Verification items for the finished model (mm, model axes). Give positions to 0.01 mm unless a question says otherwise; leave off trailing zeros. Loops run counter-clockwise (first coordinate to the right, second up) from the corner with the lowest first, then second, coordinate; pieces in that order, holes last. Notation, with made-up numbers: (40, 49) - (53, 49) arc R34 cw to (53, 81) - close; hole circle Ø1 at (26.25, 89). An arc over 180 degrees is marked (long way). Use one line per item in the form item = value.
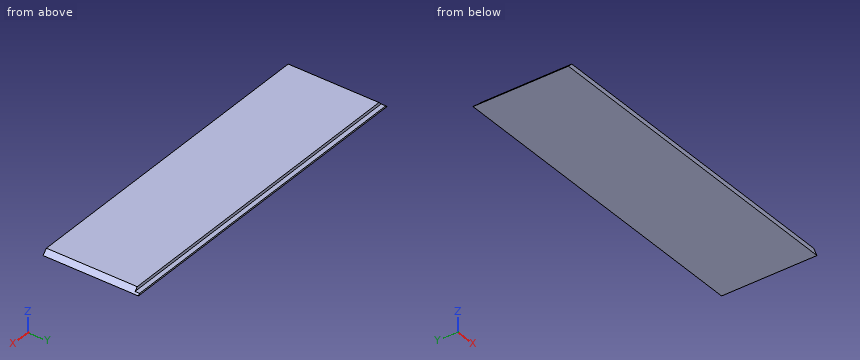
```python
from build123d import *

# Parameters (mm, degrees)
F0_W     = 1450
F0_H     = 415
F1_DEPTH = 20
F2_W     = 20
F2_H     = 13
F3_DEPTH = 1450
F5_DEPTH = 510


with BuildPart() as f1:
    # F0 (on Top) → F1 (new body)
    with BuildSketch(Plane.XY):
        Rectangle(F0_W, F0_H)
    extrude(amount=F1_DEPTH)

    # F2 (on face) → F3 (cut)
    with BuildSketch(Plane.YZ.offset(725)):
        with Locations((197.5, 13.5)):
            Rectangle(F2_W, F2_H)
    extrude(amount=-F3_DEPTH, mode=Mode.SUBTRACT)

    # F4 (on face) → F5 (cut)
    with BuildSketch(Plane.XZ.offset(207.5)):
        Polygon((725, 0), (725, 20), (705, 20), align=None)
        Polygon((-725, 20), (-725, 0), (-705, 20), align=None)
    extrude(amount=-F5_DEPTH, mode=Mode.SUBTRACT)


solid = f1.part
```
1. Depth check by flat-ended pin: pin 1 Ø5 at (y, z) = (139.5, 4) entering from -X; pin 2 Ø6 at (x, z) = (-21.5, 12.5) entering from +Y; pin 3 Ø2 at (y, z) = (-135.5, 7.5) entering from -X. Enter the tip coordinate at first touch or a pass-through.
Result set:
pin_1 = -723.5
pin_2 = 187.5
pin_3 = -718.5
2. Section check A-A, the plane x = 37. Record the cut outline in (y, z).
Result set:
outline = (-207.5, 0) - (207.5, 0) - (207.5, 7) - (187.5, 7) - (187.5, 20) - (-207.5, 20) - close
3. Scan lines: probe 1 along Y at (x, z) = (-551, 17); probe 2 along X at (y, z) = (129, 7); probe 3 along X at (y, z) = (-170, 8.75). Record each from-to range of solid material in increasing order.
Result set:
probe_1 = -207.5 to 187.5
probe_2 = -718 to 718
probe_3 = -716.25 to 716.25
4. Section check B-B, the plane z = 14. Record the cut outline in (x, y).
Result set:
outline = (-711, -207.5) - (711, -207.5) - (711, 187.5) - (-711, 187.5) - close
